```python
from build123d import *

# Parameters (mm, degrees)
SKETCH1_W           = 7
SKETCH1_H           = 12
BOSS_EXTRUDE1_DEPTH = 6
SKETCH2_R           = 3
SKETCH2_R_2         = 1.9
BOSS_EXTRUDE2_DEPTH = 2.5
SKETCH3_R           = 0.5
BOSS_EXTRUDE3_DEPTH = 1
SKETCH4_W           = 2.7
SKETCH4_H           = 2
SKETCH4_W_2         = 2
SKETCH4_H_2         = 3.1
BOSS_EXTRUDE4_DEPTH = 0.1


with BuildPart() as part:
    # Sketch1 → Boss-Extrude1 (new body)
    with BuildSketch(Plane.XY):
        Rectangle(SKETCH1_W, SKETCH1_H)
    extrude(amount=BOSS_EXTRUDE1_DEPTH)

    # Sketch2 → Boss-Extrude2 (add)
    with BuildSketch(Plane.XZ.offset(6)):
        with Locations(Location((0, 3, 0), (0, 0, 270))):
            Circle(SKETCH2_R)
        with Locations(Location((0, 3, 0), (0, 0, 270))):
            Circle(SKETCH2_R_2, mode=Mode.SUBTRACT)
    extrude(amount=BOSS_EXTRUDE2_DEPTH)

    # Sketch3 → Boss-Extrude3 (add)
    with BuildSketch(Plane(origin=(0, 0, 0), x_dir=(-1, 0, 0), z_dir=(0, 0, -1))):
        with Locations(Location((0, -4, 0), (0, 0, 180))):
            Circle(SKETCH3_R)
        with Locations(Location((0, 3, 0), (0, 0, 180))):
            Circle(SKETCH3_R)
    extrude(amount=BOSS_EXTRUDE3_DEPTH)

    # Sketch4 → Boss-Extrude4 (add, symmetric)
    with BuildSketch(Plane(origin=(0, 0, 0), x_dir=(-1, 0, 0), z_dir=(0, 0, -1))):
        with Locations((3.85, 5.5)):
            Rectangle(SKETCH4_W, SKETCH4_H)
        with Locations((3.85, -2.5)):
            Rectangle(SKETCH4_W, SKETCH4_H)
        with Locations((0, 6.55)):
            Rectangle(SKETCH4_W_2, SKETCH4_H_2)
        with Locations((-3.85, -2.5)):
            Rectangle(SKETCH4_W, SKETCH4_H)
        with Locations((-3.85, 5.5)):
            Rectangle(SKETCH4_W, SKETCH4_H)
    extrude(amount=BOSS_EXTRUDE4_DEPTH, both=True)


solid = part.part
```
The model under review builds one solid part; all positions refer to its coordinate system, in mm. A direction names the side the tool comes from. Give positions to 0.01 mm unless a question says otherwise; leave off trailing zeros. Loops run counter-clockwise (first coordinate to the right, second up) from the corner with the lowest first, then second, coordinate; pieces in that order, holes last. Notation, with made-up numbers: (52, 71) - (79, 71) arc R7 ccw to (79, 78) - close; hole circle Ø11 at (39, -13.75). An arc over 180 degrees is marked (long way). Answer as a JSON object with one key per item and string values.
Q1. For faces 1 (the cylindrical face through (2.03, -7.23, 5.21)), 2 (the flat face through (4, -2, 0.1)), 3 (the flat face through (0, 7, 0.1)), list the 3-axis set-ups (+Z, -Z, +X, -X, +Y, -Y) from which the entire face can be reached by the end or side of a thin tool; tool diameter is ignored.
Worked out:
{"face 1": "-Y", "face 2": "+Z, +X, +Y, -Y", "face 3": "+Z, +X, -X, +Y"}
Q2. To check wall thickness, follow line 1 along Y through (x, z) = (-4.25, 0); line 2 along X through (y, z) = (-5.75, 1.25); line 3 along Y through (x, z) = (2.75, 1.5). State the ranges of each line that lie inside material, in increasing order.
Worked out:
{"line 1": "y = -3.5 to -1.5, 4.5 to 6.5", "line 2": "x = -3.5 to 3.5", "line 3": "y = -6 to 6"}
Q3. Add section B-B on y = 3. State the section outline as (x, z) points, plus the area to 3 significant figures.
Worked out:
{"outline": "(-3.5, 0) - (-0.5, 0) - (-0.5, -1) - (0.5, -1) - (0.5, 0) - (3.5, 0) - (3.5, 6) - (-3.5, 6) - close", "area": "43.0 mm^2"}
Q4. Insertion check: pin 1 (0.6 mm diameter, centred on x = -4, y = -2.5, fed in from -Z); pin 2 (1.9 mm diameter, centred on x = 0, z = 3.5, fed in from -Y); pin 3 (1 mm diameter, centred on x = 0.5, z = 3, fed in from +Y); pin 4 (1.5 mm diameter, centred on x = 3, z = 4, fed in from -Y). Each pin has a flat end and moves straight along its axis. Give the tip position at first contact, or say it passes through.
Worked out:
{"pin 1": "stops at z = -0.1", "pin 2": "stops at y = -6", "pin 3": "stops at y = 6", "pin 4": "stops at y = -8.5"}
Q5. Add section C-C on z = 5.75. State the section outline as (x, y) points.
Worked out:
{"outline": "(-3.5, -6) - (-1.2, -6) - (-1.2, -8.5) - (1.2, -8.5) - (1.2, -6) - (3.5, -6) - (3.5, 6) - (-3.5, 6) - close"}
Q6. Mouldability with a two-part tool opening along Y and no side actions: class faces 4 (the flat face through (3.2, -6, 2.8)), 5 (the flat face through (0, 0, 0)), 6 (the flat face through (4, 6, -0.1)), 7 (the cylindrical face through (-0.065, -4.496, -0.493)) as +Y half, -Y half, draft (parallel to the pull), parting line (faces both ways), or undercut.
Worked out:
{"face 4": "-Y half", "face 5": "undercut", "face 6": "draft", "face 7": "undercut"}
Q7. Add section D-D on y = -2.5. State the section outline as (x, z) points, plus the area to 3 significant figures.
Worked out:
{"outline": "(-5.2, -0.1) - (-2.5, -0.1) - (-2.5, 0) - (2.5, 0) - (2.5, -0.1) - (5.2, -0.1) - (5.2, 0.1) - (3.5, 0.1) - (3.5, 6) - (-3.5, 6) - (-3.5, 0.1) - (-5.2, 0.1) - close", "area": "42.9 mm^2"}
Q8. Add section A-A on x = 4.75. State the section outline as (y, z) points.
Worked out:
{"outline": "(-3.5, -0.1) - (-1.5, -0.1) - (-1.5, 0.1) - (-3.5, 0.1) - close; (4.5, -0.1) - (6.5, -0.1) - (6.5, 0.1) - (4.5, 0.1) - close"}
